Source: CAD feature listing. Evaluate the final solid. Frame: model axes, mm. Coordinates: 2 decimals unless noted, no trailing zeros. Write each loop counter-clockwise with the first axis right and the second up, starting at its lowest first coordinate (ties: lowest second). Pieces come first, ordered by that corner, then holes. Notation, with made-up numbers: (62.25, 10) -> (89.25, 10) arc R20 cw to (89.25, 41) -> close; hole circle Ø1 at (0, -11). An arc over 180 degrees is marked (long way). One line per item, written item: value. Start each with the question number.
1. Line query: line 1 (Z direction, x = 15.5, y = 0.4); line 2 (X direction, y = 3.2, z = -44); line 3 (Z direction, x = 20, y = 3.75). Output: solid intervals per line, ascending.
2. Section query B-B, the plane x = 55. Output: boundary loops of the cut face in (y, z).
3. Section query D-D, the plane z = -26. Output: boundary loops of the cut face in (x, y), and give its area (3 significant figures).
4. Section query C-C, the plane x = 31. Output: boundary loops of the cut face in (y, z), and give its area (3 significant figures).
5. Mould query, pull axis X, two halves, no side actions, for faces 1 (the flat face through (0, 3, -30)), 2 (the flat face through (60, 3, -30)), 3 (the flat face through (30, 3, -60)), 4 (the cylindrical face through (14.185, 2.958, -18.04)). Classes: released by +X, released by -X, zero draft, split by the parting line, or undercut.
6. Section query A-A, the plane z = -5. Output: boundary loops of the cut face in (x, y).
from build123d import *

# Parameters (mm, degrees)
SKETCH1_W           = 60
SKETCH1_H           = 60
SKETCH1_R           = 2.75
SKETCH1_R_2         = 17
BOSS_EXTRUDE1_DEPTH = 6
SKETCH3_R           = 3
CUT_EXTRUDE1_DEPTH  = 10


with BuildPart() as part:
    # Sketch1 → Boss-Extrude1 (new body)
    with BuildSketch(Plane(origin=(0, 0, 0), x_dir=(1, 0, 0), z_dir=(0, 1, 0))):
        with Locations((30, 30)):
            Rectangle(SKETCH1_W, SKETCH1_H)
        with Locations(Location((15.857864376, 44.142135624, 0), (0, 0, 270))):
            Circle(SKETCH1_R, mode=Mode.SUBTRACT)
        with Locations(Location((30, 30, 0), (0, 0, 270))):
            Circle(SKETCH1_R_2, mode=Mode.SUBTRACT)
        with Locations(Location((44.142135624, 44.142135624, 0), (0, 0, 270))):
            Circle(SKETCH1_R, mode=Mode.SUBTRACT)
        with Locations(Location((44.142135624, 15.857864376, 0), (0, 0, 270))):
            Circle(SKETCH1_R, mode=Mode.SUBTRACT)
        with Locations(Location((15.857864376, 15.857864376, 0), (0, 0, 270))):
            Circle(SKETCH1_R, mode=Mode.SUBTRACT)
    extrude(amount=BOSS_EXTRUDE1_DEPTH)

    # Sketch3 → Cut-Extrude1 (cut)
    with BuildSketch(Plane(origin=(0, 6, 0), x_dir=(1, 0, 0), z_dir=(0, 1, 0))):
        with Locations(Location((5, 55, 0), (0, 0, 270))):
            Circle(SKETCH3_R)
        with Locations(Location((55, 55, 0), (0, 0, 270))):
            Circle(SKETCH3_R)
        with Locations(Location((55, 5, 0), (0, 0, 270))):
            Circle(SKETCH3_R)
        with Locations(Location((5, 5, 0), (0, 0, 270))):
            Circle(SKETCH3_R)
    extrude(amount=-CUT_EXTRUDE1_DEPTH, mode=Mode.SUBTRACT)


solid = part.part
Computed values:
1. line 1: z = -60 to -46.87, -41.42 to -38.87, -21.13 to -18.58, -13.13 to 0
1. line 2: x = 0 to 13.11, 18.6 to 20.36, 39.64 to 41.4, 46.89 to 60
1. line 3: z = -60 to -43.75, -16.25 to 0
2. outline: (0, -60) -> (6, -60) -> (6, -58) -> (0, -58) -> close; (0, -52) -> (6, -52) -> (6, -8) -> (0, -8) -> close; (0, -2) -> (6, -2) -> (6, 0) -> (0, 0) -> close
3. outline: (0, 0) -> (13.48, 0) -> (13.48, 6) -> (0, 6) -> close; (46.52, 0) -> (60, 0) -> (60, 6) -> (46.52, 6) -> close
3. area: 162 mm²
4. outline: (0, -60) -> (6, -60) -> (6, -46.97) -> (0, -46.97) -> close; (0, -13.03) -> (6, -13.03) -> (6, 0) -> (0, 0) -> close
4. area: 156 mm²
5. face 1: released by -X
5. face 2: released by +X
5. face 3: zero draft
5. face 4: undercut
6. outline: (0, 0) -> (2, 0) -> (2, 6) -> (0, 6) -> close; (8, 0) -> (52, 0) -> (52, 6) -> (8, 6) -> close; (58, 0) -> (60, 0) -> (60, 6) -> (58, 6) -> close
